Part model, mm, in its own coordinate system. A direction names the side the tool comes from. Round coordinates to 2 decimals unless told otherwise and drop trailing zeros. Order: outer loops, then holes, each group sorted by start corner. A loop starts at its lowest first (then second) coordinate and runs counter-clockwise, first axis right, second up. Notation, with made-up numbers: M 60,16 L 68,16 A19 cw 68,36 Z; hole C 45.25,85 d3. An arc over 180 degrees is marked long. Write each question's results on one line, items separated by ' | '. Start each with the question number.
1. Band-saw the part on A-A, the plane x = 4. List the corners of the cut face in (y, z), then the cut area to 3 significant figures.
2. Drop flat-ended pins along their axis: pin 1 Ø1.5 at (x, z) = (2.5, 5.5) entering from +Y; pin 2 Ø3.5 at (x, y) = (5, 9.5) entering from +Z. Give the stop position or say it passes through.
3. Band-saw the part on B-B, the plane y = 9.75. List the corners of the cut face in (x, z), then the cut area to 3 significant figures.
4. Which spindle directions (+Z, -Z, +X, -X, +Y, -Y) get a long thin tool onto all of the face, cutting with end or side? Do faces 1 (the face through (8, 15, 1)), 2 (the face through (7, 9, 2)). Say none if no direction does.
5. Probe L1, parallel to Y at x = 4.25, z = 3.5; L2, parallel to Y at x = 10, z = 2.25. List the from-to ranges inside material, lowest first. Write a range as [from, to].
Autodesk Fusion 360 part; units mm, degrees
sketch "Sketch1" plane through (0, 0, 0) normal (0, 0, 1) x (1, 0, 0)
  line L0 (0, 0) -> (15, 0)
  line L1 (15, 0) -> (15, 15)
  line L2 (15, 15) -> (0, 15)
  line L3 (0, 15) -> (0, 0)
  dimension "d1" = 15
  dimension "d2" = 15
extrude "Extrude1" add sketch "Sketch1" along normal blind 2
sketch "Sketch2" plane through (0, 0, 2) normal (0, 0, 1) x (-1, 0, 0)
  line L0 (0, -15) -> (0, 0)
  line L1 (0, 0) -> (-15, 0)
  line L2 (-15, 0) -> (-15, -15)
  line L3 (-15, -15) -> (0, -15)
  line L4 (0, 0) -> (-15, 0)
  line L5 (-15, 0) -> (-15, -2)
  line L6 (-15, -2) -> (0, -2)
  line L7 (0, -2) -> (0, 0)
  dimension "d5" = 2
extrude "Extrude2" add sketch "Sketch2" along normal blind 13 contours L0 L1 L2 L4 L5 L6 L7
chamfer "Chamfer1" distance 1 angle 45 1 edges at (7.5, 2, 2)
Solution:
1) outline: M 0,0 L 15,0 L 15,2 L 3,2 L 2,3 L 2,15 L 0,15 Z | area: 56.5 mm^2
2) pin 1: y = 2 | pin 2: z = 2
3) outline: M 0,0 L 15,0 L 15,2 L 0,2 Z | area: 30.0 mm^2
4) face 1: +Z, -Z, +X, -X, +Y | face 2: +Z, +X, -X, +Y
5) L1: [0, 2] | L2: [0, 2.75]
